from build123d import *

# Parameters (mm, degrees)
SKETCH1_R           = 6.1
SKETCH1_R_2         = 1.6
BOSS_EXTRUDE1_DEPTH = 7.4
SKETCH2_R           = 1.8
CUT_EXTRUDE2_DEPTH  = 4
SKETCH3_R           = 1.2
CUT_EXTRUDE3_DEPTH  = 1
SKETCH4_R           = 52.225
BOSS_EXTRUDE2_DEPTH = 8
FILLET1_R           = 1


with BuildPart() as part:
    # Sketch1 → Boss-Extrude1 (new body)
    # profile 1 of 3: a face of its own
    with BuildSketch(Plane(origin=(0, 0, 0), x_dir=(1, 0, 0), z_dir=(0, 1, 0))):
        Circle(SKETCH1_R)
        with Locations(Location((0, 0, 0), (0, 0, 270))):
            Circle(SKETCH1_R_2, mode=Mode.SUBTRACT)
    # profile 2 of 3: a face of its own
    with BuildSketch(Plane(origin=(0, 0, 0), x_dir=(1, 0, 0), z_dir=(0, 1, 0))):
        with BuildLine():
            ThreePointArc((0, -6.1), (-4.313351365, -4.313351365), (-6.1, 0))
            Line((-6.1, 0), (-6.1, -6.1))
            Line((-6.1, -6.1), (0, -6.1))
        make_face()
    # profile 3 of 3: a face of its own
    with BuildSketch(Plane(origin=(0, 0, 0), x_dir=(1, 0, 0), z_dir=(0, 1, 0))):
        with BuildLine():
            ThreePointArc((-6.1, 0), (-4.313351365, 4.313351365), (0, 6.1))
            Line((0, 6.1), (-6.1, 6.1))
            Line((-6.1, 6.1), (-6.1, 0))
        make_face()
    extrude(amount=BOSS_EXTRUDE1_DEPTH)

    # Sketch2 → Cut-Extrude2 (cut)
    with BuildSketch(Plane.ZY.offset(6.1)):
        with Locations((0, 3.7)):
            Circle(SKETCH2_R)
    extrude(amount=-CUT_EXTRUDE2_DEPTH, mode=Mode.SUBTRACT)

    # Sketch3 → Cut-Extrude3 (cut)
    with BuildSketch(Plane.ZY.offset(2.1)):
        with Locations((0, 3.7)):
            Circle(SKETCH3_R)
    extrude(amount=-CUT_EXTRUDE3_DEPTH, mode=Mode.SUBTRACT)

    # Sketch4 → Boss-Extrude2 (add)
    with BuildSketch(Plane(origin=(0, 7.4, 0), x_dir=(1, 0, 0), z_dir=(0, 1, 0))):
        with Locations(Location((0, 0, 0), (0, 0, 270))):
            Circle(SKETCH4_R)
    extrude(amount=BOSS_EXTRUDE2_DEPTH)

    # Sketch6 → Cut-Revolve1 (revolve, cut)
    with BuildSketch(Plane(origin=(0, 0, 0), x_dir=(0, 0, -1), z_dir=(1, 0, 0)), mode=Mode.PRIVATE) as cut_revolve1_sk:
        Polygon((-46.225, 11.4), (-50.225, 7.4), (-52.225, 7.4), (-52.225, 15.4), (-50.225, 15.4), align=None)
    revolve(cut_revolve1_sk.sketch.rotate(Axis((0, 0, 0), (0, 1, 0)), 180), axis=Axis((0, 0, 0), (0, 1, 0)), mode=Mode.SUBTRACT)

    # Fillet1
    fillet1_edges = [part.edges().sort_by_distance(p)[0] for p in [
        (6.1, 7.4, 0),
        (-3.05, 7.4, -6.1),
        (-6.1, 7.4, 0),
        (-3.05, 7.4, 6.1),
    ]]
    fillet(fillet1_edges, radius=FILLET1_R)


solid = part.part
Here's how the part is built. I have some questions about the finished solid (model axes, mm). A direction names the side the tool comes from. Coordinates: 2 decimals unless noted, no trailing zeros. Order: outer loops, then holes, each group sorted by start corner. A loop starts at its lowest first (then second) coordinate and runs counter-clockwise, first axis right, second up. Notation, with made-up numbers: (31.25, 33.5) - (78.25, 33.5) arc R21 ccw to (78.25, 40.5) - close; hole circle Ø10 at (-35.5, 82). An arc over 180 degrees is marked (long way). Use CSV: the item, a comma, the result in double quotes. Start each with the question number.
1. I'm going to push flat-ended pins straight in: pin 1 (4 mm diameter, centred on y = 3, z = -1, fed in from -X); pin 2 (6 mm diameter, centred on x = -30, z = -38, fed in from -Y); pin 3 (1 mm diameter, centred on y = 5, z = 34, fed in from +X); pin 4 (3 mm diameter, centred on x = -2, y = 3, fed in from +Z). Where does each tip first touch, or does it pass through?
2. Please list where these lines run through material, in increasing order: line 1 (Y direction, x = -3.7, z = 0); line 2 (Z direction, x = -1.5, y = 3.7); line 3 (X direction, y = 3.5, z = 0). Write a range as from..to.
3. If we mould it in two halves opening along X, with no side actions, what happens to faces 6 (the face through (-46.08, 11.15, 6.05)), 7 (the face through (1.586, 3.648, -0.208)), 8 (the face through (-3, 3, 6.1))? For each: +X half, -X half, draft (parallel to the pull), parting line (faces both ways), or undercut.
4. Suppose I cut it at B-B on y = 13. List the corners of the cut face in (x, z) for me (3 decimals).
5. For faces 1 (the face through (6.1, 3.2, 0.1)), 2 (the face through (28.245, 11.594, 36.837)), 3 (the face through (-3, 3, -6.1)), 4 (the face through (0, 7.4, 0)), 5 (the face through (-1.72, 4.71, 0.65)), which set-ups out of +Z, -Z, +X, -X, +Y, -Y let a thin tool reach every point of the face, with its end or its side?
6. Suppose I cut it at A-A on z = 0. List the corners of the cut face in (x, y) for me (3 decimals), then the cut area to 3 significant figures.
Output:
1,pin 1,"stops at x = -6.1"
1,pin 2,"stops at y = 7.4"
1,pin 3,"passes through"
1,pin 4,"stops at z = 6.1"
2,line 1,"y = 0..1.9, 5.5..15.4"
2,line 2,"z = -6.1..-1.2, 1.2..6.1"
2,line 3,"x = 1.6..6.1"
3,face 6,"parting line"
3,face 7,"undercut"
3,face 8,"draft"
4,outline,"circle Ø95.65 at (0, 0)"
5,face 1,"+X, -Y"
5,face 2,"none"
5,face 3,"-Z, +X, -X, -Y"
5,face 4,"-Y"
5,face 5,"-X"
6,outline,"(-50.225, 7.4) - (-7.1, 7.4) arc R1 cw to (-6.1, 6.4) - (-6.1, 5.5) - (-2.1, 5.5) - (-2.1, 4.9) - (-1.6, 4.9) - (-1.6, 7.4) - (1.6, 7.4) - (1.6, 0) - (6.1, 0) - (6.1, 6.4) arc R1 cw to (7.1, 7.4) - (50.225, 7.4) - (46.225, 11.4) - (50.225, 15.4) - (-50.225, 15.4) - (-46.225, 11.4) - close; (-6.1, 0) - (-1.6, 0) - (-1.6, 2.5) - (-2.1, 2.5) - (-2.1, 1.9) - (-6.1, 1.9) - close"
6,area,"823 mm2"
